Study the drawing (mm; zero at the part's minimum x, y, z) and answer. A direction names the side the tool comes from. Coordinates: 2 decimals unless noted, no trailing zeros. Order: outer loops, then holes, each group sorted by start corner. A loop starts at its lowest first (then second) coordinate and runs counter-clockwise, first axis right, second up. Notation, with made-up numbers: (-13, -19.5) -> (29, -19.5) arc R26 ccw to (29, 9.5) -> close; hole circle Ø1 at (22, 53.5). An arc over 180 degrees is marked (long way). Answer as CSV lines item,"result". Start each with the question number.
Item 1: For a pull along X with two mould halves and no side action, classify the marked faces 1, 2 and 3 as pulls with the +X half, pulls with the -X half, needs draft (parallel to the pull), parting line crosses it, or undercut.
Item 2: Which of the six approach directions +Z, -Z, +X, -X, +Y, -Y give full straight-line access (tool end or side, diameter ignored) to the marked faces 4, 5 and 6?
Item 3: Section B-B (z = 15) is taken. Write down the section's boundary in (x, y).
Item 4: Each of these flat-tipped pins is pushed along its axis until it touches: pin 1 Ø24 at (x, z) = (22.5, 38.5) entering from -Y; pin 2 Ø20 at (x, y) = (24.5, 18.5) entering from +Z. Where does it stop, or does it pass through?
Item 5: Section A-A (y = 15) is taken. Write down the section's boundary in (x, z).
Item 6: Section C-C (x = 28.5) is taken. Write down the section's boundary in (y, z), then the cut area to 3 significant figures.
Item 7: Section D-D (y = 22) is taken. Write down the section's boundary in (x, z), then the cut area to 3 significant figures.
Item 8: Straight lines are drawn through the part: L1, parallel to X at y = 16, z = 9; L2, parallel to Y at x = 29, z = 4; L3, parallel to Z at x = 51, y = 16.5. For each, find the intervals that lie inside material, in ascending order.
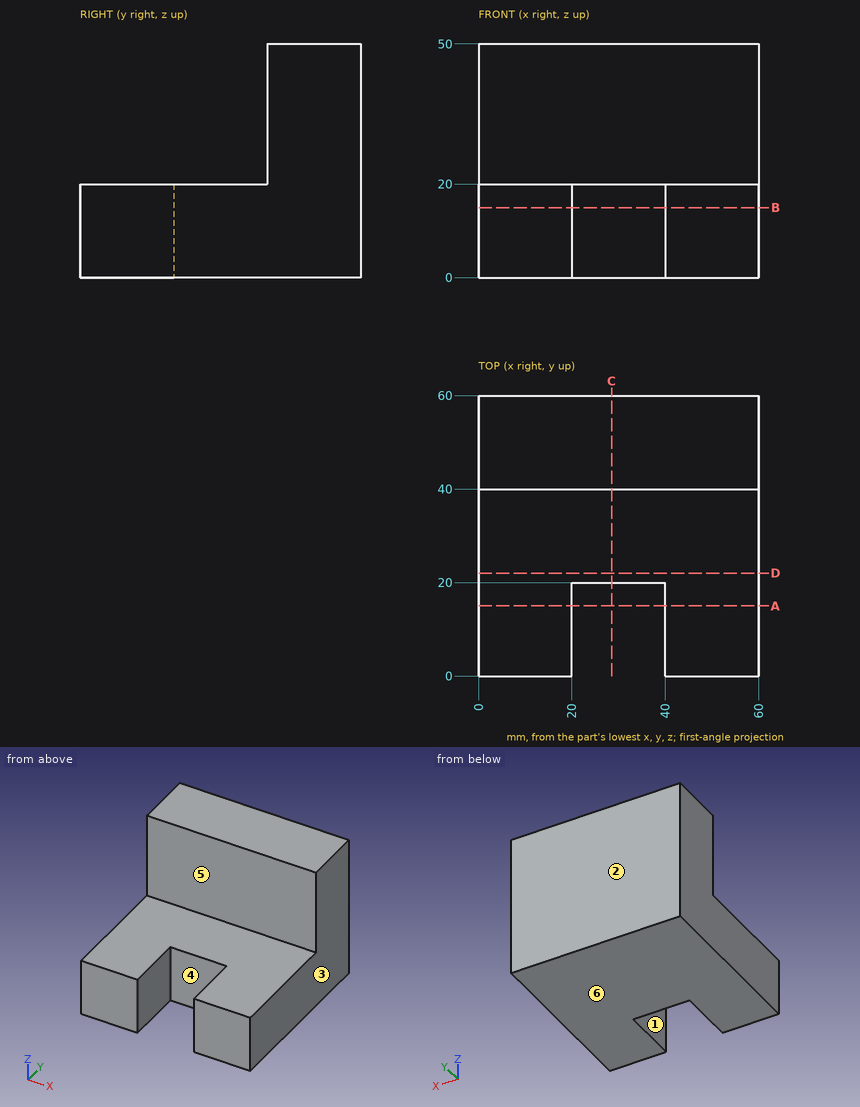
Checked values:
1,face 1,"undercut"
1,face 2,"needs draft"
1,face 3,"pulls with the +X half"
2,face 4,"+Z, -Z, -Y"
2,face 5,"+Z, +X, -X, -Y"
2,face 6,"-Z, +X, -X, +Y, -Y"
3,outline,"(0, 0) -> (20, 0) -> (20, 20) -> (40, 20) -> (40, 0) -> (60, 0) -> (60, 60) -> (0, 60) -> close"
4,pin 1,"stops at y = 40"
4,pin 2,"stops at z = 20"
5,outline,"(0, 0) -> (20, 0) -> (20, 20) -> (0, 20) -> close; (40, 0) -> (60, 0) -> (60, 20) -> (40, 20) -> close"
6,outline,"(20, 0) -> (60, 0) -> (60, 50) -> (40, 50) -> (40, 20) -> (20, 20) -> close"
6,area,"1,400 mm^2"
7,outline,"(0, 0) -> (60, 0) -> (60, 20) -> (0, 20) -> close"
7,area,"1,200 mm^2"
8,L1,"x = 0 to 20, 40 to 60"
8,L2,"y = 20 to 60"
8,L3,"z = 0 to 20"
